Part model, mm, in its own coordinate system. Give positions to 0.01 mm unless a question says otherwise; leave off trailing zeros. Loops run counter-clockwise (first coordinate to the right, second up) from the corner with the lowest first, then second, coordinate; pieces in that order, holes last. Notation, with made-up numbers: (21.25, -5.5) -> (31.25, -5.5) arc R32 ccw to (31.25, 33.5) -> close; hole circle Ø3 at (31.25, 3.25). An arc over 180 degrees is marked (long way). One line per question, with ' | ' between items.
```python
from build123d import *

# Parameters (mm, degrees)
SKETCH1_W          = 3.175
SKETCH1_H          = 268.22908
BASE_FLANGE1_DEPTH = 101.6
HEM1_START         = -268.22908
HEM1_DEPTH         = 268.22908
HEM1_2_DEPTH       = 268.22908
SKETCH10_R         = 2.45745
CUT_EXTRUDE1_DEPTH = 287.898940147
FILLET1_R          = 3.175


# Read off the part's stored shape, not the designer's step: Hem1
# Sheet-metal steps are written as plain solids
with BuildPart() as part:
    # Sketch1 → Base-Flange1 (new body)
    with BuildSketch(Plane(origin=(0, 0, 0), x_dir=(1, 0, 0), z_dir=(0, 1, 0))):
        with Locations((1.5875, 134.11454)):
            Rectangle(SKETCH1_W, SKETCH1_H)
    extrude(amount=BASE_FLANGE1_DEPTH)

    # Hem1 outline → Hem1 (cut)
    with BuildSketch(Plane.XY.offset(HEM1_START)):
        with BuildLine():
            ThreePointArc((0, 98.375), (0.926970953, 100.637672645), (3.175, 101.59961238))
            Line((3.175, 101.59961238), (3.175, 101.6))
            Line((3.175, 101.6), (0, 101.6))
            Line((0, 101.6), (0, 98.375))
        make_face()
        with BuildLine():
            ThreePointArc((3.175, 0.00038762), (0.926970953, 0.962327355), (0, 3.225))
            Line((0, 3.225), (0, 0))
            Line((0, 0), (3.175, 0))
            Line((3.175, 0), (3.175, 0.00038762))
        make_face()
    extrude(amount=HEM1_DEPTH, mode=Mode.SUBTRACT)

    # Hem1 2 outline → Hem1 2 (add)
    with BuildSketch(Plane.XY.offset(HEM1_START)):
        with BuildLine():
            Line((3.275, 88.9), (6.45, 88.9))
            Line((6.45, 88.9), (6.45, 98.375))
            ThreePointArc((6.45, 98.375), (5.487672645, 100.673029047), (3.175, 101.59961238))
            Line((3.175, 101.59961238), (3.175, 98.375))
            ThreePointArc((3.175, 98.375), (3.225, 98.425), (3.275, 98.375))
            Line((3.275, 98.375), (3.275, 88.9))
        make_face()
        with BuildLine():
            ThreePointArc((3.275, 3.225), (3.225, 3.175), (3.175, 3.225))
            Line((3.175, 3.225), (3.175, 0.00038762))
            ThreePointArc((3.175, 0.00038762), (5.487672645, 0.926970953), (6.45, 3.225))
            Line((6.45, 3.225), (6.45, 12.7))
            Line((6.45, 12.7), (3.275, 12.7))
            Line((3.275, 12.7), (3.275, 3.225))
        make_face()
    extrude(amount=HEM1_2_DEPTH)

    # Sketch10 → Cut-Extrude1 (cut, through all)
    with BuildSketch(Plane.ZY):
        with Locations((-255.52908, 76.15)):
            Circle(SKETCH10_R)
        with Locations((-255.52908, 25.35)):
            Circle(SKETCH10_R)
        with Locations((-230.12908, 25.35)):
            Circle(SKETCH10_R)
        with Locations((-230.12908, 76.15)):
            Circle(SKETCH10_R)
        with Locations((-12.7, 76.15)):
            Circle(SKETCH10_R)
        with Locations((-12.7, 25.35)):
            Circle(SKETCH10_R)
    extrude(amount=-CUT_EXTRUDE1_DEPTH, mode=Mode.SUBTRACT)

    # Fillet1
    fillet1_edges = [part.edges().sort_by_distance(p)[0] for p in [
        (4.8625, 88.9, 0),
        (4.8625, 88.9, -268.22908),
        (4.8625, 12.7, -268.22908),
        (4.8625, 12.7, 0),
    ]]
    fillet(fillet1_edges, radius=FILLET1_R)


solid = part.part
```
1) Saw through at B-B (z = -12.7). Give the cut face in (x, y) (3 decimals).
Found:
outline: (0, 3.225) arc R3.225 ccw to (6.45, 3.225) -> (6.45, 12.7) -> (3.275, 12.7) -> (3.275, 3.225) arc R0.05 cw to (3.175, 3.225) -> (3.175, 22.893) -> (0, 22.893) -> close; (0, 27.807) -> (3.175, 27.807) -> (3.175, 73.693) -> (0, 73.693) -> close; (0, 78.607) -> (3.175, 78.607) -> (3.175, 98.375) arc R0.05 cw to (3.275, 98.375) -> (3.275, 88.9) -> (6.45, 88.9) -> (6.45, 98.375) arc R3.225 ccw to (0, 98.375) -> close
2) Pull direction Z, two halves, no side cores. Call faces 1 (the cylindrical face through (1.57, 24.41, -227.86)), 2 (the flat face through (6.45, 94, -136)), 3 (the cylindrical face through (1.565, 76.888, -253.185)), 4 (the flat face through (2, 52, -268.229)): pulls with the +Z half, pulls with the -Z half, needs draft (parallel to the pull), parting line crosses it, or undercut.
Found:
face 1: undercut | face 2: needs draft | face 3: undercut | face 4: pulls with the -Z half
3) Saw through at C-C (z = -84). Give the cut face in (x, y) (3 decimals), and give its area (3 significant figures).
Found:
outline: (0, 3.225) arc R3.225 ccw to (6.45, 3.225) -> (6.45, 12.7) -> (3.275, 12.7) -> (3.275, 3.225) arc R0.05 cw to (3.175, 3.225) -> (3.175, 98.375) arc R0.05 cw to (3.275, 98.375) -> (3.275, 88.9) -> (6.45, 88.9) -> (6.45, 98.375) arc R3.225 ccw to (0, 98.375) -> close | area: 395 mm2
4) Drill centre lines: line 1 (Y direction, x = 1.9, z = -12.7); line 2 (Y direction, x = 0.85, z = -12.7); line 3 (X direction, y = 53.5, z = -229.5) (3 decimals). Where is each one in solid material? Low to high.
Found:
line 1: 0.28 to 22.89, 27.81 to 73.69, 78.61 to 101.32 | line 2: 1.04 to 22.89, 27.81 to 73.69, 78.61 to 100.56 | line 3: 0 to 3.175
5) Saw through at A-A (y = 76.15). Give the cut face in (x, z) (3 decimals), and give its area (3 significant figures).
Found:
outline: (0, -268.229) -> (3.175, -268.229) -> (3.175, -257.987) -> (0, -257.987) -> close; (0, -253.072) -> (3.175, -253.072) -> (3.175, -232.587) -> (0, -232.587) -> close; (0, -227.672) -> (3.175, -227.672) -> (3.175, -15.157) -> (0, -15.157) -> close; (0, -10.243) -> (3.175, -10.243) -> (3.175, 0) -> (0, 0) -> close | area: 805 mm2
6) Saw through at D-D (x = 5). Give the cut face in (y, z) (3 decimals).
Found:
outline: (0.532, -268.229) -> (9.525, -268.229) arc R3.175 ccw to (12.7, -265.054) -> (12.7, -3.175) arc R3.175 ccw to (9.525, 0) -> (0.532, 0) -> close; (88.9, -265.054) arc R3.175 ccw to (92.075, -268.229) -> (101.068, -268.229) -> (101.068, 0) -> (92.075, 0) arc R3.175 ccw to (88.9, -3.175) -> close
7) Pin check, flat tips, straight feed: P1, Ø8, axis at y = 76.15, z = -12.7, coming from the +X side (3 decimals); P2, Ø2.5, axis at x = 5, z = -83.5, coming from the -Y side; P3, Ø1, axis at x = 5, z = -171, coming from the +Y side. Stop position of each tip, or through.
Found:
P1: x = 3.175 | P2: y = 0.04 | P3: y = 101.34
